Design review of the part shown in the three views and the two pictorial views. Dimensions are in mm from the part's minimum x, y and z. A direction names the side the tool comes from. Coordinates: 2 decimals unless noted, no trailing zeros. Loops run counter-clockwise (first coordinate to the right, second up) from the corner with the lowest first, then second, coordinate; pieces in that order, holes last. Notation, with made-up numbers: (-14, 14.5) -> (-6, 14.5) arc R20 ccw to (-6, 21.5) -> close; hole circle Ø8 at (65, 30). An arc over 180 degrees is marked (long way). Use a Markdown table: item, result. Add a question column.
Q1. Take a section at D-D on z = 1.75. Write out the cut boundary in (x, y), plus the area to 3 significant figures.
Q2. Clearance check with flat-ended pins moving along their axes: pin 1 Ø3 at (x, z) = (22.5, 12) entering from +Y; pin 2 Ø10 at (y, z) = (23.5, 15.5) entering from +X; pin 3 Ø5 at (x, z) = (22.5, 13) entering from -Y. State where each tip first meets the part, or that it passes through.
Q3. For the marked faces 1, 2, 3, 4 and 5, list the 3-axis set-ups (+Z, -Z, +X, -X, +Y, -Y) from which the entire face can be reached by the end or side of a thin tool; tool diameter is ignored.
Q4. For probe 1 along X at (y, z) = (31.5, 11); probe 2 along Y at (x, z) = (22.25, 6.75); probe 3 along X at (y, z) = (3.5, 3), list the stretches that pass through material, from the lowest coordinate up.
Q5. Take a section at A-A on z = 15.7. Write out the cut boundary in (x, y).
Q6. Take a section at C-C on y = 28. Write out the cut boundary in (x, z), plus the area to 3 significant figures.
Q7. Take a section at B-B on x = 4.75. Write out the cut boundary in (y, z), plus the area to 3 significant figures.
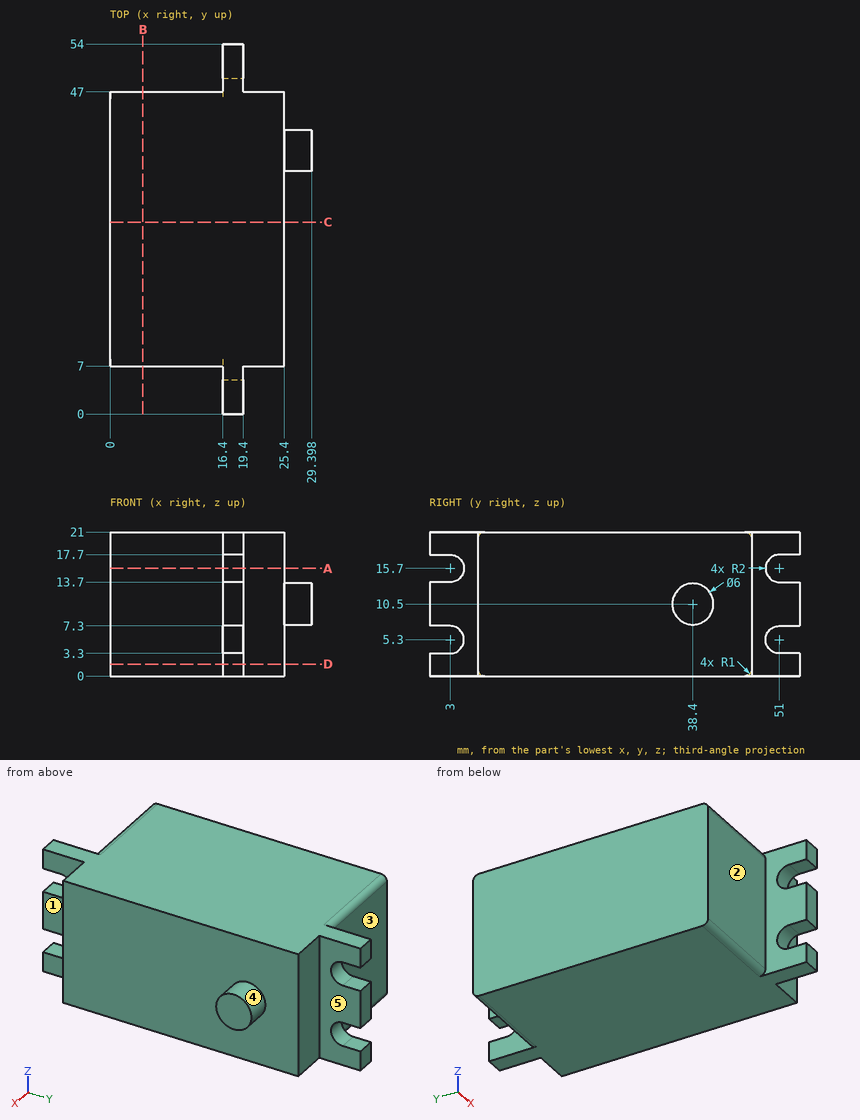
Answer list:
| question | item | result |
|---|---|---|
| 1 | outline | (0, 7) -> (16.4, 7) -> (16.4, 0) -> (19.4, 0) -> (19.4, 7) -> (25.4, 7) -> (25.4, 47) -> (19.4, 47) -> (19.4, 54) -> (16.4, 54) -> (16.4, 47) -> (0, 47) -> close |
| 1 | area | 1,060 mm² |
| 2 | pin 1 | y = 47 |
| 2 | pin 2 | x = 25.4 |
| 2 | pin 3 | y = 7 |
| 3 | face 1 | +Z, -Z, +X, -Y |
| 3 | face 2 | +Z, -Z, -X, -Y |
| 3 | face 3 | +Z, -Z, -X, +Y |
| 3 | face 4 | +X |
| 3 | face 5 | +Z, -Z, +X, +Y |
| 4 | probe 1 | 0 to 25.4 |
| 4 | probe 2 | 7 to 47 |
| 4 | probe 3 | 16.4 to 19.4 |
| 5 | outline | (0, 7) -> (16.4, 7) -> (16.4, 5) -> (19.4, 5) -> (19.4, 7) -> (25.4, 7) -> (25.4, 47) -> (19.4, 47) -> (19.4, 49) -> (16.4, 49) -> (16.4, 47) -> (0, 47) -> close |
| 6 | outline | (0, 0) -> (25.4, 0) -> (25.4, 21) -> (0, 21) -> close |
| 6 | area | 533 mm² |
| 7 | outline | (7, 1) arc R1 ccw to (8, 0) -> (46, 0) arc R1 ccw to (47, 1) -> (47, 20) arc R1 ccw to (46, 21) -> (8, 21) arc R1 ccw to (7, 20) -> close |
| 7 | area | 839 mm² |
